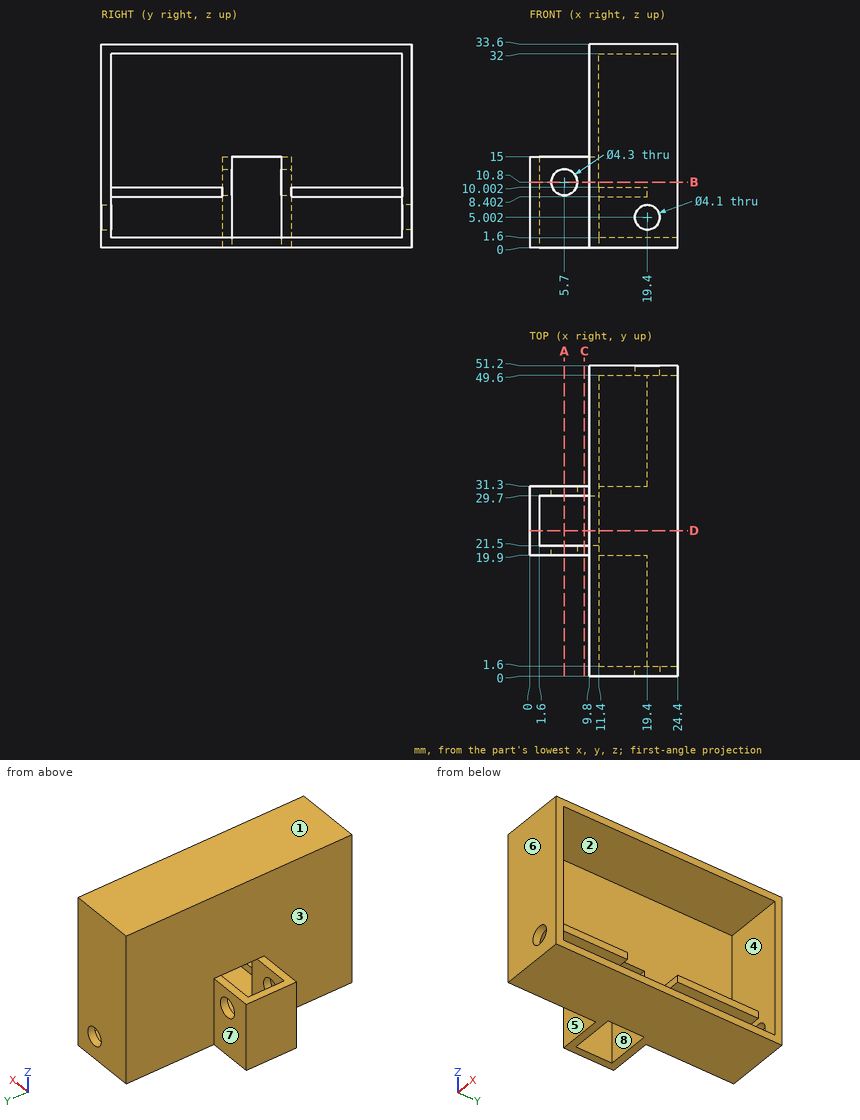
Source: three-view drawing plus pictorial views. Frame: mm from the lowest corner of the part. A direction names the side the tool comes from. Give positions to 0.01 mm unless a question says otherwise; leave off trailing zeros. Order: outer loops, then holes, each group sorted by start corner. A loop starts at its lowest first (then second) coordinate and runs counter-clockwise, first axis right, second up. Notation, with made-up numbers: (87.5, 31.5) -> (127.5, 31.5) arc R20 ccw to (127.5, 48.5) -> close; hole circle Ø4 at (45.25, 85.25). An arc over 180 degrees is marked (long way). Write each question's results on one line, items separated by ' | '. Start each with the question number.
Item 1: Set-up query: the marked faces 4, 5, 6, 7 and 8. Return all of +Z, -Z, +X, -X, +Y, -Y with unobstructed straight access to the full face (end or side cutting, diameter ignored); none if empty.
Item 2: Line query: line 1 (Z direction, x = 16.5, y = 43.5); line 2 (Y direction, x = 14.5, z = 5); line 3 (Z direction, x = 22, y = 12). Output: solid intervals per line, ascending.
Item 3: Cut plane C-C on x = 9. Return the cut outline in (y, z), then the cut area to 3 significant figures.
Item 4: Mould query, pull axis Z, two halves, no side actions, for the marked faces 1, 2 and 3. Classes: pulls with the +Z half, pulls with the -Z half, needs draft (parallel to the pull), parting line crosses it, or undercut.
Item 5: Cut plane D-D on y = 24. Return the cut outline in (x, z).
Item 6: Cut plane A-A on x = 5.7. Return the cut outline in (y, z).
Item 7: Cut plane B-B on z = 10.8. Return the cut outline in (x, y).
Item 8: Contact query for flat-ended pins moving along their axis: P1, Ø3, axis at x = 6.5, z = 9, coming from the -Y side; P2, Ø1.5, axis at x = 4, z = 9, coming from the +Y side; P3, Ø3.5, axis at x = 19.4, z = 5, coming from the +Y side; P4, Ø4, axis at y = 26.5, z = 8, coming from the +X side. Output: stop coordinate, or through.
Established:
1) face 4: +X | face 5: +Z, -Z, -X, -Y | face 6: +Z, -Z, +X, -X, -Y | face 7: +Z, -Z, -X, +Y | face 8: -Z
2) line 1: 0 to 1.6, 8.4 to 10, 32 to 33.6 | line 2: 0 to 1.6, 49.6 to 51.2 | line 3: 0 to 1.6, 32 to 33.6
3) outline: (19.9, 0) -> (21.5, 0) -> (21.5, 15) -> (19.9, 15) -> close; (29.7, 0) -> (31.3, 0) -> (31.3, 15) -> (29.7, 15) -> close | area: 48.0 mm^2
4) face 1: pulls with the +Z half | face 2: undercut | face 3: needs draft
5) outline: (0, 0) -> (1.6, 0) -> (1.6, 15) -> (0, 15) -> close; (9.8, 15) -> (11.4, 15) -> (11.4, 32) -> (24.4, 32) -> (24.4, 33.6) -> (9.8, 33.6) -> close; (11.4, 0) -> (24.4, 0) -> (24.4, 1.6) -> (11.4, 1.6) -> close
6) outline: (19.9, 0) -> (21.5, 0) -> (21.5, 8.65) -> (19.9, 8.65) -> close; (19.9, 12.95) -> (21.5, 12.95) -> (21.5, 15) -> (19.9, 15) -> close; (29.7, 0) -> (31.3, 0) -> (31.3, 8.65) -> (29.7, 8.65) -> close; (29.7, 12.95) -> (31.3, 12.95) -> (31.3, 15) -> (29.7, 15) -> close
7) outline: (0, 19.9) -> (3.55, 19.9) -> (3.55, 21.5) -> (1.6, 21.5) -> (1.6, 29.7) -> (3.55, 29.7) -> (3.55, 31.3) -> (0, 31.3) -> close; (7.85, 19.9) -> (9.8, 19.9) -> (9.8, 0) -> (24.4, 0) -> (24.4, 1.6) -> (11.4, 1.6) -> (11.4, 21.5) -> (7.85, 21.5) -> close; (7.85, 29.7) -> (11.4, 29.7) -> (11.4, 49.6) -> (24.4, 49.6) -> (24.4, 51.2) -> (9.8, 51.2) -> (9.8, 31.3) -> (7.85, 31.3) -> close
8) P1: y = 19.9 | P2: y = 31.3 | P3: through | P4: x = 1.6
